Design review of the part built by this model. Coordinates are the model's own, in mm. Face numbers are marked on the shaded views. A direction names the side the tool comes from. Coordinates: 2 decimals unless noted, no trailing zeros. Loops run counter-clockwise (first coordinate to the right, second up) from the corner with the lowest first, then second, coordinate; pieces in that order, holes last. Notation, with made-up numbers: (-27, 59) - (17, 59) arc R31 cw to (17, 87) - close; hole circle Ø11 at (8.5, 51.5). An arc over 180 degrees is marked (long way). Use one line per item in the form item = value. Start each with the question number.
(1) For L1, parallel to Z at x = 45.5, y = 21.5; L2, parallel to Y at x = -23, z = 16.5; L3, parallel to Y at x = -12, z = 18.5, list the stretches that pass through material, from the lowest coordinate up.
(2) Add section C-C (x = 42). State the section outline as (y, z) points.
(3) The part is to be moulded in two halves that separate along Z. For the marked faces 1, 2 and 3, say which applies: pulls with the +Z half, pulls with the -Z half, needs draft (parallel to the pull), parting line crosses it, or undercut.
(4) Add section D-D (y = -3). State the section outline as (x, z) points, plus the area to 3 significant figures.
(5) Clearance check with flat-ended pins moving along their axes: pin 1 Ø9.5 at (x, y) = (25, -29) entering from +Z; pin 2 Ø3 at (x, z) = (-25.5, 12) entering from +Y; pin 3 Ø8 at (y, z) = (8.5, 34) entering from -X; pin 4 Ø3 at (x, y) = (28, -24) entering from -Z. State where each tip first meets the part, or that it passes through.
(6) Tool access review of the marked faces 4, 5, 6, 7 and 8: name each direction out of +Z, -Z, +X, -X, +Y, -Y from which nothing blocks a thin tool from reaching the whole face with its end or side.
(7) Add section A-A (z = 38). State the section outline as (x, y) points, plus the area to 3 significant figures.
(8) Add section B-B (x = 31). State the section outline as (y, z) points.
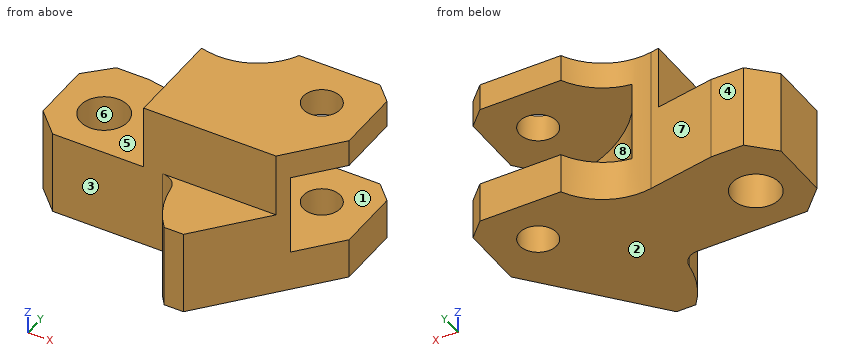
```python
from build123d import *

# Parameters (mm, degrees)
F0_R     = 7
F0_R_2   = 5.5
F1_DEPTH = 44
F2_R     = 7
F3_DEPTH = 19
F5_R     = 41
F6_DEPTH = 24
F8_DEPTH = 19


with BuildPart() as f1:
    # F0 (on Top) → F1 (new body)
    with BuildSketch(Plane.XY):
        with BuildLine():
            Line((-20.4506443609, 16.7664520695), (-30.0882231277, 16.7664520695))
            Line((-30.0882231277, 16.7664520695), (-37.0882231277, 9.7664520695))
            Line((-37.0882231277, 9.7664520695), (-37.0882231277, -8.2335479305))
            Line((-37.0882231277, -8.2335479305), (-30.0882231277, -15.2335479305))
            Line((-30.0882231277, -15.2335479305), (2.4873157836, -15.2335479305))
            ThreePointArc((2.4873157836, -15.2335479305), (5.7525515647, -16.4469616983), (7.432954525, -19.4982538128))
            ThreePointArc((7.432954525, -19.4982538128), (9.7697847282, -27.3492199915), (14.208756925, -34.2335479305))
            Line((14.208756925, -34.2335479305), (19.9117768723, -34.2335479305))
            Line((19.9117768723, -34.2335479305), (48.9117768723, -0.2335479305))
            Line((48.9117768723, -0.2335479305), (48.9117768723, 18.7664520695))
            Line((48.9117768723, 18.7664520695), (43.9117768723, 23.7664520695))
            Line((43.9117768723, 23.7664520695), (19.9117768723, 23.7664520695))
            ThreePointArc((19.9117768723, 23.7664520695), (11.4619798371, 15.0687874681), (-0.5277319739, 13.2535050814))
            Line((-0.5277319739, 13.2535050814), (-20.4506443609, 16.7664520695))
        make_face()
        with Locations((-23.0882231277, -1.2335479305)):
            Circle(F0_R, mode=Mode.SUBTRACT)
        with Locations((34.9117768723, 9.7664520695)):
            Circle(F0_R_2, mode=Mode.SUBTRACT)
    extrude(amount=F1_DEPTH)

    # F2 (on face) → F3 (cut)
    with BuildSketch(Plane.XY.offset(44)):
        Polygon((-30.0882231277, -15.2335479305), (-3.0882231277, -15.2335479305), (-3.0882231277, 13.7049887557), (-20.4506443609, 16.7664520695), (-30.0882231277, 16.7664520695), (-37.0882231277, 9.7664520695), (-37.0882231277, -8.2335479305), align=None)
        with Locations((-23.0882231277, -1.2335479305)):
            Circle(F2_R, mode=Mode.SUBTRACT)
    extrude(amount=-F3_DEPTH, mode=Mode.SUBTRACT)

    # F5 (on offset) → F6 (cut)
    with BuildSketch(Plane.XY.offset(36)):
        with Locations((43.189617951, 28.5173000447)):
            Circle(F5_R)
    extrude(amount=-F6_DEPTH, mode=Mode.SUBTRACT)

    # F7 (on face) → F8 (cut)
    with BuildSketch(Plane.XY.offset(44)):
        with BuildLine():
            Line((36.1176592252, -15.2335479305), (2.4873157836, -15.2335479305))
            ThreePointArc((2.4873157836, -15.2335479305), (5.7525515647, -16.4469616983), (7.432954525, -19.4982538128))
            ThreePointArc((7.432954525, -19.4982538128), (9.7697847282, -27.3492199915), (14.208756925, -34.2335479305))
            Line((14.208756925, -34.2335479305), (19.9117768723, -34.2335479305))
            Line((19.9117768723, -34.2335479305), (36.1176592252, -15.2335479305))
        make_face()
    extrude(amount=-F8_DEPTH, mode=Mode.SUBTRACT)


solid = f1.part
```
Computed values:
q1.L1 = 0 to 12, 36 to 44
q1.L2 = -15.23 to -8.23, 5.77 to 16.77
q1.L3 = -15.23 to 15.28
q2.outline = (-8.34, 0) - (23.77, 0) - (23.77, 12) - (-8.34, 12) - close; (-8.34, 36) - (23.77, 36) - (23.77, 44) - (-8.34, 44) - close
q3.face_1 = undercut
q3.face_2 = pulls with the -Z half
q3.face_3 = needs draft
q4.outline = (-37.09, 0) - (-29.86, 0) - (-29.86, 25) - (-37.09, 25) - close; (-16.31, 0) - (46.55, 0) - (46.55, 12) - (16.97, 12) - (16.97, 36) - (46.55, 36) - (46.55, 44) - (-3.09, 44) - (-3.09, 25) - (-16.31, 25) - close
q4.area = 1,990 mm^2
q5.pin_1 = 25
q5.pin_2 = 16.77
q5.pin_3 = -3.09
q5.pin_4 = 0
q6.face_4 = +Z, -Z, -X, +Y
q6.face_5 = +Z, -X, +Y, -Y
q6.face_6 = +Z, -Z
q6.face_7 = +Z, -Z, +Y
q6.face_8 = +X, +Y
q7.outline = (-3.09, -15.23) - (36.12, -15.23) - (48.91, -0.23) - (48.91, 18.77) - (43.91, 23.77) - (19.91, 23.77) arc R19 cw to (-0.53, 13.25) - (-3.09, 13.7) - close; hole circle Ø11 at (34.91, 9.77)
q7.area = 1,630 mm^2
q8.outline = (-21.23, 0) - (5.9, 0) - (5.9, 12) - (-10.63, 12) - (-10.63, 36) - (5.9, 36) - (5.9, 44) - (-15.23, 44) - (-15.23, 25) - (-21.23, 25) - close; (13.63, 0) - (23.77, 0) - (23.77, 12) - (13.63, 12) - close; (13.63, 36) - (23.77, 36) - (23.77, 44) - (13.63, 44) - close
